Verification items for the finished model (mm, model axes). Face numbers are marked on the shaded views. A direction names the side the tool comes from. Coordinates: 2 decimals unless noted, no trailing zeros. Write each loop counter-clockwise with the first axis right and the second up, starting at its lowest first coordinate (ties: lowest second). Pieces come first, ordered by that corner, then holes. Notation, with made-up numbers: (33, 81) -> (84, 81) arc R22 ccw to (84, 114) -> close; hole circle Ø5 at (63.25, -12.75). An arc over 180 degrees is marked (long way). Answer in a Markdown table with one row per item.
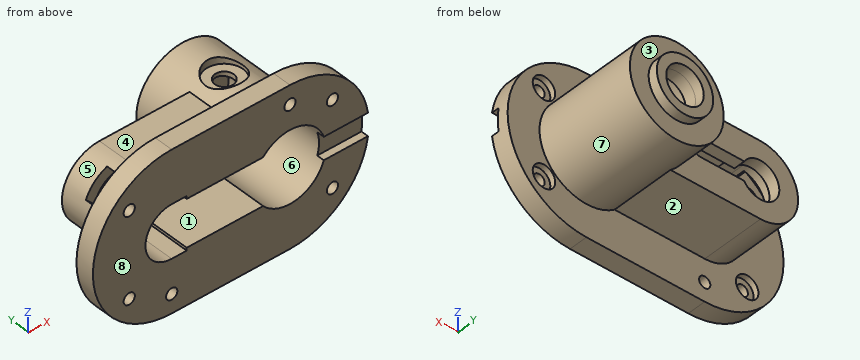
```python
from build123d import *
from build123d.topology import SkipClean

# Parameters (mm, degrees)
EXTRUDE_1_DEPTH                       = 10
SKETCH_2_R                            = 6
SKETCH_2_R_2                          = 3
CUT_EXTRUDE_1_DEPTH                   = 3
SKETCH_2_2_R                          = 3
CUT_EXTRUDE_2_DEPTH                   = 86.242301705
EXTRUDE_2_DEPTH                       = 34
SKETCH_3_3_R                          = 25
EXTRUDE_3_DEPTH                       = 55
SHELL_START                           = 10
SHELL_9_DEPTH                         = 28
SHELL_START_2                         = 38
SHELL_9_2_OUTLINE_R                   = 19
SHELL_9_2_DEPTH                       = 21
SKETCH_5_R                            = 19
CUT_EXTRUDE_5_DEPTH                   = 10
SKETCH_6_R                            = 10
CUT_EXTRUDE_6_DEPTH                   = 6
SKETCH_7_R                            = 15
SKETCH_7_R_2                          = 10
EXTRUDE_4_DEPTH                       = 5
CUT_EXTRUDE_START                     = 25
SKETCH_8_R                            = 10
SKETCH_8_R_2                          = 5
CUT_EXTRUDE_7_DEPTH                   = 4
SKETCH_8_2_R                          = 5
CUT_EXTRUDE_8_DEPTH                   = 110.846483785
SKETCH_9_R                            = 10
CUT_EXTRUDE_9_DEPTH                   = 6
EXTRUDE_START                         = -14
SKETCH_10_W                           = 42.154767421
SKETCH_10_H                           = 38
EXTRUDE_5_DEPTH                       = 1.5
EXTRUDE_START_2                       = 14
SKETCH_10_2_W                         = 42.154767421
SKETCH_10_2_H                         = 38
EXTRUDE_6_DEPTH                       = 1.5
SKETCH_11_R                           = 19
CUT_EXTRUDE_10_DEPTH                  = 104.185512549
CUT_EXTRUDE_START_2                   = 49.527756
SKETCH_12_W                           = 12
SKETCH_12_H                           = 4
CUT_EXTRUDE_11_DEPTH                  = 23.972244
SKETCH_13_R                           = 3
CUT_EXTRUDE_13_DEPTH                  = 110.846483785
CUT_EXTRUDE_14_REACH                  = 141.071
CUT_EXTRUDE_14_END_RADIUS             = 14
SKETCH_15_W                           = 16
SKETCH_15_H                           = 16
CUT_EXTRUDE_14_DIRECTION_2_REACH      = 141.071
CUT_EXTRUDE_14_DIRECTION_2_END_RADIUS = 20


# Read off the part's stored shape, not the designer's step: the shell step
with BuildPart() as part:
    # Sketch 1 → Extrude 1 (new body)
    with BuildSketch(Plane(origin=(0, 0, 0), x_dir=(1, 0, 0), z_dir=(0, 1, 0))):
        with BuildLine():
            Line((-31.5, 42), (31.5, 42))
            ThreePointArc((31.5, 42), (73.5, 0), (31.5, -42))
            Line((31.5, -42), (-31.5, -42))
            ThreePointArc((-31.5, -42), (-73.5, 0), (-31.5, 42))
        make_face()
    extrude(amount=EXTRUDE_1_DEPTH)

    # Sketch 2 → Cut-Extrude 1 (cut)
    # profile 1 of 4: a face of its own
    with BuildSketch(Plane(origin=(0, 10, 0), x_dir=(1, 0, 0), z_dir=(0, 1, 0))):
        with Locations(Location((54.127416998, 22.627416998, 0), (0, 0, 270))):
            Circle(SKETCH_2_R)
        with Locations(Location((54.127416998, 22.627416998, 0), (0, 0, 270))):
            Circle(SKETCH_2_R_2, mode=Mode.SUBTRACT)
    # profile 2 of 4: a face of its own
    with BuildSketch(Plane(origin=(0, 10, 0), x_dir=(1, 0, 0), z_dir=(0, 1, 0))):
        with Locations(Location((54.127416998, -22.627416998, 0), (0, 0, 90))):
            Circle(SKETCH_2_R)
        with Locations(Location((54.127416998, -22.627416998, 0), (0, 0, 90))):
            Circle(SKETCH_2_R_2, mode=Mode.SUBTRACT)
    # profile 3 of 4: a face of its own
    with BuildSketch(Plane(origin=(0, 10, 0), x_dir=(1, 0, 0), z_dir=(0, 1, 0))):
        with Locations(Location((-54.127416998, -22.627416998, 0), (0, 0, 270))):
            Circle(SKETCH_2_R)
        with Locations(Location((-54.127416998, -22.627416998, 0), (0, 0, 270))):
            Circle(SKETCH_2_R_2, mode=Mode.SUBTRACT)
    # profile 4 of 4: a face of its own
    with BuildSketch(Plane(origin=(0, 10, 0), x_dir=(1, 0, 0), z_dir=(0, 1, 0))):
        with Locations(Location((-54.127416998, 22.627416998, 0), (0, 0, 90))):
            Circle(SKETCH_2_R)
        with Locations(Location((-54.127416998, 22.627416998, 0), (0, 0, 90))):
            Circle(SKETCH_2_R_2, mode=Mode.SUBTRACT)
    extrude(amount=-CUT_EXTRUDE_1_DEPTH, mode=Mode.SUBTRACT)

    # Sketch 2_2 → Cut-Extrude 2 (cut, through all)
    with BuildSketch(Plane(origin=(0, 10, 0), x_dir=(1, 0, 0), z_dir=(0, 1, 0))):
        with Locations(Location((-54.127416998, -22.627416998, 0), (0, 0, 270))):
            Circle(SKETCH_2_2_R)
        with Locations(Location((-54.127416998, 22.627416998, 0), (0, 0, 270))):
            Circle(SKETCH_2_2_R)
        with Locations(Location((54.127416998, 22.627416998, 0), (0, 0, 270))):
            Circle(SKETCH_2_2_R)
        with Locations(Location((54.127416998, -22.627416998, 0), (0, 0, 270))):
            Circle(SKETCH_2_2_R)
    extrude(amount=-CUT_EXTRUDE_2_DEPTH, mode=Mode.SUBTRACT)

    # Sketch 5 → Cut-Extrude 5 (cut)
    with BuildSketch(Plane(origin=(0, 0, 0), x_dir=(1, 0, 0), z_dir=(0, 1, 0))):
        with Locations(Location((31.5, 0, 0), (0, 0, 132.536898363))):
            Circle(SKETCH_5_R)
        with BuildLine():
            Line((18.654767421, -14), (-31.5, -14))
            ThreePointArc((-31.5, -14), (-45.5, 0), (-31.5, 14))
            Line((-31.5, 14), (18.654767421, 14))
            ThreePointArc((18.654767421, 14), (12.5, 0), (18.654767421, -14))
        make_face()
    extrude(amount=CUT_EXTRUDE_5_DEPTH, mode=Mode.SUBTRACT)



with BuildPart() as body_2:
    # Sketch 3 → Extrude 2 (new body)
    with BuildSketch(Plane(origin=(0, 10, 0), x_dir=(1, 0, 0), z_dir=(0, 1, 0))):
        with BuildLine():
            Line((16.5, 20), (-31.5, 20))
            ThreePointArc((-31.5, 20), (-51.5, 0), (-31.5, -20))
            Line((-31.5, -20), (16.5, -20))
            ThreePointArc((16.5, -20), (6.5, 0), (16.5, 20))
        make_face()
    extrude(amount=EXTRUDE_2_DEPTH)


with BuildPart() as body_3:
    # Sketch 3_3 → Extrude 3 (new body)
    with BuildSketch(Plane(origin=(0, 10, 0), x_dir=(1, 0, 0), z_dir=(0, 1, 0))):
        with Locations(Location((31.5, 0, 0), (0, 0, 270))):
            Circle(SKETCH_3_3_R)
    extrude(amount=EXTRUDE_3_DEPTH)


with BuildPart() as body_2_1:
    add(body_2.part)

    # Combine 1: union body 3
    add(body_3.part)

    # Shell 9 outline → Shell 9 (cut)
    with BuildSketch(Plane(origin=(0, 0, 0), x_dir=(1, 0, 0), z_dir=(0, 1, 0)).offset(SHELL_START)):
        with BuildLine():
            Line((-31.5, -14), (18.654767421, -14))
            ThreePointArc((18.654767421, -14), (50.5, 0), (18.654767421, 14))
            Line((18.654767421, 14), (-31.5, 14))
            ThreePointArc((-31.5, 14), (-45.5, 0), (-31.5, -14))
        make_face()
    extrude(amount=SHELL_9_DEPTH, mode=Mode.SUBTRACT)

    # Shell 9 2 outline → Shell 9 2 (cut)
    with BuildSketch(Plane(origin=(0, 0, 0), x_dir=(1, 0, 0), z_dir=(0, 1, 0)).offset(SHELL_START_2)):
        with Locations((31.5, 0)):
            Circle(SHELL_9_2_OUTLINE_R)
    extrude(amount=SHELL_9_2_DEPTH, mode=Mode.SUBTRACT)

    # Sketch 6 → Cut-Extrude 6 (cut)
    with BuildSketch(Plane.XZ.offset(-59)):
        with Locations(Location((31.5, 0, 0), (0, 0, 270))):
            Circle(SKETCH_6_R)
    extrude(amount=-CUT_EXTRUDE_6_DEPTH, mode=Mode.SUBTRACT)

    # Sketch 7 → Extrude 4 (add)
    with BuildSketch(Plane(origin=(0, 65, 0), x_dir=(1, 0, 0), z_dir=(0, 1, 0))):
        with Locations(Location((31.5, 0, 0), (0, 0, 270))):
            Circle(SKETCH_7_R)
        with Locations(Location((31.5, 0, 0), (0, 0, 90))):
            Circle(SKETCH_7_R_2, mode=Mode.SUBTRACT)
    extrude(amount=EXTRUDE_4_DEPTH)

    # Sketch 8 → Cut-Extrude 7 (cut)
    with BuildSketch(Plane.XY.offset(CUT_EXTRUDE_START)):
        with Locations((31.5, 40)):
            Circle(SKETCH_8_R)
        with Locations((31.5, 40)):
            Circle(SKETCH_8_R_2, mode=Mode.SUBTRACT)
    extrude(amount=-CUT_EXTRUDE_7_DEPTH, mode=Mode.SUBTRACT)

    # Sketch 8_2 → Cut-Extrude 8 (cut, through all)
    with BuildSketch(Plane.XY):
        with Locations(Location((31.5, 40, 0), (0, 0, 180))):
            Circle(SKETCH_8_2_R)
    extrude(amount=CUT_EXTRUDE_8_DEPTH, mode=Mode.SUBTRACT)

    # Sketch 9 → Cut-Extrude 9 (cut)
    with BuildSketch(Plane(origin=(0, 44, 0), x_dir=(1, 0, 0), z_dir=(0, 1, 0))):
        with Locations((-31.5, 0)):
            Circle(SKETCH_9_R)
        with BuildLine():
            Line((-31.5, 5), (0.5, 5))
            ThreePointArc((0.5, 5), (5.5, 0), (0.5, -5))
            Line((0.5, -5), (-31.5, -5))
            ThreePointArc((-31.5, -5), (-36.5, 0), (-31.5, 5))
        make_face()
    extrude(amount=-CUT_EXTRUDE_9_DEPTH, mode=Mode.SUBTRACT)


with BuildPart() as part_1:
    add(part.part)

    add(body_2_1.part)  # Extrude 5 merges body 2
    # Sketch 10 → Extrude 5 (add)
    with BuildSketch(Plane.XY.offset(EXTRUDE_START)):
        with Locations((-2.422616289, 19)):
            Rectangle(SKETCH_10_W, SKETCH_10_H)
    extrude(amount=EXTRUDE_5_DEPTH)

    # Sketch 10_2 → Extrude 6 (add)
    with BuildSketch(Plane.XY.offset(EXTRUDE_START_2)):
        with Locations((-2.422616289, 19)):
            Rectangle(SKETCH_10_2_W, SKETCH_10_2_H)
    extrude(amount=-EXTRUDE_6_DEPTH)

    # Sketch 11 → Cut-Extrude 10 (cut, through all)
    with SkipClean():  # the faces are left unmerged after this step: merging them gives an invalid solid
        with BuildSketch(Plane.XZ.offset(-59)):
            with Locations(Location((31.5, 0, 0), (0, 0, 221.139510415))):
                Circle(SKETCH_11_R)
        extrude(amount=CUT_EXTRUDE_10_DEPTH, mode=Mode.SUBTRACT)

    # Sketch 12 → Cut-Extrude 11 (cut)
    with SkipClean():  # the faces are left unmerged after this step: merging them gives an invalid solid
        with BuildSketch(Plane(origin=(0, 0, 0), x_dir=(0, 0, -1), z_dir=(1, 0, 0)).offset(CUT_EXTRUDE_START_2)):
            with Locations((0, 2)):
                Rectangle(SKETCH_12_W, SKETCH_12_H)
        extrude(amount=CUT_EXTRUDE_11_DEPTH, mode=Mode.SUBTRACT)

    # Sketch 13 → Cut-Extrude 13 (cut, through all)
    with SkipClean():  # the faces are left unmerged after this step: merging them gives an invalid solid
        with BuildSketch(Plane(origin=(0, 0, 0), x_dir=(1, 0, 0), z_dir=(0, 1, 0))):
            with Locations(Location((-31.5, 32, 0), (0, 0, 270))):
                Circle(SKETCH_13_R)
            with Locations(Location((31.5, -32, 0), (0, 0, 270))):
                Circle(SKETCH_13_R)
        extrude(amount=CUT_EXTRUDE_13_DEPTH, mode=Mode.SUBTRACT)

    # Cut-Extrude 14: up to this cylinder (the profile starts outside it)
    with SkipClean():  # the faces are left unmerged after this step: merging them gives an invalid solid
        cut_extrude_14_end = Plane(origin=(-31.5, 23, 0), z_dir=(0, -1, 0)) * Cylinder(CUT_EXTRUDE_14_END_RADIUS, 311.142, mode=Mode.PRIVATE)
        # Sketch 15 → Cut-Extrude 14 (cut, up to the surface)
        with BuildSketch(Plane(origin=(-25.75, 0, 25.75), x_dir=(0, -1, 0), z_dir=(-0.7071067811865488, 0, 0.7071067811865464)), mode=Mode.PRIVATE) as cut_extrude_14_sk1:
            with Locations((-23, -22.273863607)):
                Rectangle(SKETCH_15_W, SKETCH_15_H)
        cut_extrude_14_tool1 = extrude(cut_extrude_14_sk1.sketch, amount=-CUT_EXTRUDE_14_REACH, mode=Mode.PRIVATE) - cut_extrude_14_end
        add(cut_extrude_14_tool1.solids().sort_by_distance((-41.5, 23, 10))[0], mode=Mode.SUBTRACT)

    # Cut-Extrude 14 direction 2: up to this cylinder (the profile starts inside it)
    with SkipClean():  # the faces are left unmerged after this step: merging them gives an invalid solid
        cut_extrude_14_direction_2_end = Plane(origin=(-31.5, 23, 0), z_dir=(0, -1, 0)) * Cylinder(CUT_EXTRUDE_14_DIRECTION_2_END_RADIUS, 323.142, mode=Mode.PRIVATE)
        # Sketch 15 → Cut-Extrude 14 direction 2 (cut, up to the surface)
        with BuildSketch(Plane(origin=(-25.75, 0, 25.75), x_dir=(0, -1, 0), z_dir=(-0.7071067811865488, 0, 0.7071067811865464)), mode=Mode.PRIVATE) as cut_extrude_14_direction_2_sk1:
            with Locations((-23, -22.273863607)):
                Rectangle(SKETCH_15_W, SKETCH_15_H)
        cut_extrude_14_direction_2_tool1 = extrude(cut_extrude_14_direction_2_sk1.sketch, amount=CUT_EXTRUDE_14_DIRECTION_2_REACH, mode=Mode.PRIVATE) & cut_extrude_14_direction_2_end
        add(cut_extrude_14_direction_2_tool1.solids().sort_by_distance((-41.5, 23, 10))[0], mode=Mode.SUBTRACT)


solid = part_1.part
```
1. Sectioned sample at C-C, the plane z = -32. Record the cut outline in (x, y).
Findings below:
| item | result |
|---|---|
| outline | (-58.7, 0) -> (-34.5, 0) -> (-34.5, 10) -> (-58.7, 10) -> close; (-28.5, 0) -> (58.7, 0) -> (58.7, 10) -> (-28.5, 10) -> close |
2. Release check for a two-part mould opening along Z. For the marked faces 6, 7 and 8 record: released by +Z, released by -Z, zero draft, split by the parting line, or undercut.
Findings below:
| item | result |
|---|---|
| face 6 | undercut |
| face 7 | split by the parting line |
| face 8 | zero draft |
3. Sectioned sample at B-B, the plane y = 23. Record the cut outline in (x, z), and give its area (3 significant figures).
Findings below:
| item | result |
|---|---|
| outline | (-50.12, 7.3) arc R20 ccw to (-31.5, -20) -> (16.5, -20) arc R25 ccw (long way) to (16.5, 20) -> (-31.5, 20) arc R20 ccw to (-38.8, 18.62) -> (-33.97, 13.78) arc R14 cw to (-31.5, 14) -> (-23.5, 14) -> (-23.5, 12.5) -> (17.19, 12.5) arc R19 cw (long way) to (17.19, -12.5) -> (-23.5, -12.5) -> (-23.5, -14) -> (-31.5, -14) arc R14 cw to (-45.28, 2.47) -> close |
| area | 1,530 mm² |
4. Material ranges on probe 1 along X at (y, z) = (36, -1); probe 2 along Y at (x, z) = (34, 38); probe 3 along Y at (x, z) = (-14.5, -8), recorded low to high. Write a range as from..to.
Findings below:
| item | result |
|---|---|
| probe 1 | x = -51.47..-45.46, 50.47..56.48 |
| probe 2 | y = 0..10 |
| probe 3 | y = 38..44 |
5. Go/stop test with flat-tipped pins: pin 1 (8.5 mm diameter, centred on x = -5, z = 6.5, fed in from -Y); pin 2 (18 mm diameter, centred on x = -40.5, z = 12.5, fed in from +Y); pin 3 (2 mm diameter, centred on x = -39, y = 43.5, fed in from -Z). Record where each tip stops, or that it passes through.
Findings below:
| item | result |
|---|---|
| pin 1 | stops at y = 38 |
| pin 2 | stops at y = 44 |
| pin 3 | stops at z = -18.91 |
6. Sectioned sample at A-A, the plane x = -14. Record the cut outline in (y, z).
Findings below:
| item | result |
|---|---|
| outline | (0, -42) -> (10, -42) -> (10, -20) -> (44, -20) -> (44, -5) -> (38, -5) -> (38, -12.5) -> (0, -12.5) -> close; (0, 12.5) -> (38, 12.5) -> (38, 5) -> (44, 5) -> (44, 20) -> (10, 20) -> (10, 42) -> (0, 42) -> close |
7. Sectioned sample at D-D, the plane y = 40. Record the cut outline in (x, z), and give its area (3 significant figures).
Findings below:
| item | result |
|---|---|
| outline | (-31.5, -20) -> (16.5, -20) arc R25 ccw (long way) to (41.5, 22.91) -> (41.5, 21) -> (36.5, 21) -> (36.5, 18.33) arc R19 cw (long way) to (26.5, 18.33) -> (26.5, 21) -> (21.5, 21) -> (21.5, 22.91) arc R25 ccw to (16.5, 20) -> (-31.5, 20) arc R20 ccw to start; hole (-22.84, -5) -> (0.5, -5) arc R5 ccw to (0.5, 5) -> (-22.84, 5) arc R10 ccw (long way) to start |
| area | 2,430 mm² |
8. Access from +Z, -Z, +X, -X, +Y, -Y to the whole of each face (thin tool, end or side, straight path). Record for the marked faces 1, 2, 3, 4 and 5.
Findings below:
| item | result |
|---|---|
| face 1 | -Y |
| face 2 | -Z, -X, +Y |
| face 3 | +Y |
| face 4 | +Z, -X, +Y |
| face 5 | -X, +Y |
